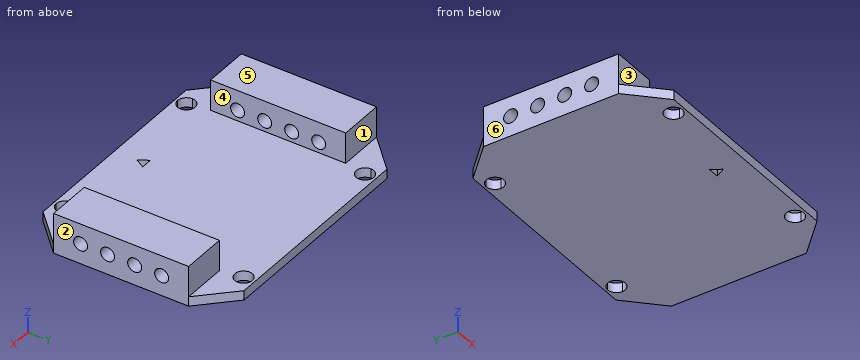
from build123d import *

# Parameters (mm, degrees)
F1_DEPTH = 1.7
F2_W     = 8.1
F2_H     = 24.2000000085
F3_DEPTH = 5.5
F6_DEPTH = 8.1
F7_DEPTH = 8.1


with BuildPart() as f1:
    # F0 (on Top) → F1 (new body)
    with BuildSketch(Plane.XY):
        with BuildLine():
            ThreePointArc((-17.5750000042, 16), (-17.1136931846, 17.1136931804), (-16.0000000042, 17.575))
            Line((-16.0000000042, 17.575), (-16.0000000042, 18))
            Line((-16.0000000042, 18), (-18.8500000085, 18))
            Line((-18.8500000085, 18), (-20.8500000085, 16))
            Line((-20.8500000085, 16), (-17.5750000042, 16))
        make_face()
        with BuildLine():
            ThreePointArc((-16.0000000042, 17.575), (-14.8863068239, 17.1136931804), (-14.4250000042, 16))
            ThreePointArc((-14.4250000042, 16), (-16.0000000042, 14.425), (-17.5750000042, 16))
            Line((-17.5750000042, 16), (-20.8500000085, 16))
            Line((-20.8500000085, 16), (-24.75, 12.1000000085))
            Line((-24.75, 12.1000000085), (-24.75, -12.1))
            Line((-24.75, -12.1), (-20.85, -16))
            Line((-20.85, -16), (-17.5749999958, -16))
            ThreePointArc((-17.5749999958, -16), (-15.9999999958, -14.425), (-14.4249999958, -16))
            ThreePointArc((-14.4249999958, -16), (-14.8863068154, -17.1136931804), (-15.9999999958, -17.575))
            Line((-15.9999999958, -17.575), (-15.9999999958, -18))
            Line((-15.9999999958, -18), (16.0000000042, -18))
            Line((16.0000000042, -18), (16.0000000042, -17.575))
            ThreePointArc((16.0000000042, -17.575), (14.8863068239, -14.8863068196), (17.5750000042, -16))
            Line((17.5750000042, -16), (20.8500000085, -16))
            Line((20.8500000085, -16), (24.75, -12.1000000085))
            Line((24.75, -12.1000000085), (24.75, 12.1))
            Line((24.75, 12.1), (20.85, 16))
            Line((20.85, 16), (17.5749999958, 16))
            ThreePointArc((17.5749999958, 16), (14.8863068154, 14.8863068196), (15.9999999958, 17.575))
            Line((15.9999999958, 17.575), (15.9999999958, 18))
            Line((15.9999999958, 18), (-16.0000000042, 18))
            Line((-16.0000000042, 18), (-16.0000000042, 17.575))
        make_face()
        Polygon((1, -12.2679491924), (0, -14), (-1, -12.2679491924), align=None, mode=Mode.SUBTRACT)
        with BuildLine():
            Line((18.85, 18), (15.9999999958, 18))
            Line((15.9999999958, 18), (15.9999999958, 17.575))
            ThreePointArc((15.9999999958, 17.575), (17.1136931761, 17.1136931804), (17.5749999958, 16))
            Line((17.5749999958, 16), (20.85, 16))
            Line((20.85, 16), (18.85, 18))
        make_face()
        with BuildLine():
            Line((18.8500000085, -18), (20.8500000085, -16))
            Line((20.8500000085, -16), (17.5750000042, -16))
            ThreePointArc((17.5750000042, -16), (17.1136931846, -17.1136931804), (16.0000000042, -17.575))
            Line((16.0000000042, -17.575), (16.0000000042, -18))
            Line((16.0000000042, -18), (18.8500000085, -18))
        make_face()
        with BuildLine():
            Line((-17.5749999958, -16), (-20.85, -16))
            Line((-20.85, -16), (-18.85, -18))
            Line((-18.85, -18), (-15.9999999958, -18))
            Line((-15.9999999958, -18), (-15.9999999958, -17.575))
            ThreePointArc((-15.9999999958, -17.575), (-17.1136931761, -17.1136931804), (-17.5749999958, -16))
        make_face()
    extrude(amount=F1_DEPTH)

    # F2 (on face) → F3 (join)
    with BuildSketch(Plane.XY.offset(1.7)):
        with Locations((-20.7, 4.2e-09)):
            Rectangle(F2_W, F2_H)
        with Locations((20.7, -4.2e-09)):
            Rectangle(F2_W, F2_H)
    extrude(amount=F3_DEPTH)

    # F5 (on face) → F6 (cut)
    with BuildSketch(Plane.YZ.offset(24.75)):
        with BuildLine():
            Line((6.0099999915, 3.6), (8.5099999915, 3.6))
            ThreePointArc((8.5099999915, 3.6), (7.2599999915, 4.85), (6.0099999915, 3.6))
        make_face()
        with BuildLine():
            ThreePointArc((6.0099999915, 3.6), (7.2599999915, 2.35), (8.5099999915, 3.6))
            Line((8.5099999915, 3.6), (6.0099999915, 3.6))
        make_face()
        with BuildLine():
            ThreePointArc((1.1699999915, 3.6), (2.4199999915, 2.35), (3.6699999915, 3.6))
            Line((3.6699999915, 3.6), (1.1699999915, 3.6))
        make_face()
        with BuildLine():
            Line((1.1699999915, 3.6), (3.6699999915, 3.6))
            ThreePointArc((3.6699999915, 3.6), (2.4199999915, 4.85), (1.1699999915, 3.6))
        make_face()
        with BuildLine():
            ThreePointArc((-3.6700000085, 3.6), (-2.4200000085, 2.35), (-1.1700000085, 3.6))
            Line((-1.1700000085, 3.6), (-3.6700000085, 3.6))
        make_face()
        with BuildLine():
            Line((-3.6700000085, 3.6), (-1.1700000085, 3.6))
            ThreePointArc((-1.1700000085, 3.6), (-2.4200000085, 4.85), (-3.6700000085, 3.6))
        make_face()
        with BuildLine():
            Line((-6.0100000085, 3.6), (-8.5100000085, 3.6))
            ThreePointArc((-8.5100000085, 3.6), (-7.2600000085, 2.35), (-6.0100000085, 3.6))
        make_face()
        with BuildLine():
            ThreePointArc((-6.0100000085, 3.6), (-7.2600000085, 4.85), (-8.5100000085, 3.6))
            Line((-8.5100000085, 3.6), (-6.0100000085, 3.6))
        make_face()
    extrude(amount=-F6_DEPTH, mode=Mode.SUBTRACT)

    # F4 (on face) → F7 (cut)
    with BuildSketch(Plane(origin=(-24.75, 0, 0), x_dir=(0, -1, 0), z_dir=(-1, 0, 0))):
        with BuildLine():
            Line((6.0099999915, 3.6), (8.5099999915, 3.6))
            ThreePointArc((8.5099999915, 3.6), (7.2599999915, 4.85), (6.0099999915, 3.6))
        make_face()
        with BuildLine():
            ThreePointArc((6.0099999915, 3.6), (7.2599999915, 2.35), (8.5099999915, 3.6))
            Line((8.5099999915, 3.6), (6.0099999915, 3.6))
        make_face()
        with BuildLine():
            Line((1.1699999915, 3.6), (3.6699999915, 3.6))
            ThreePointArc((3.6699999915, 3.6), (2.4199999915, 4.85), (1.1699999915, 3.6))
        make_face()
        with BuildLine():
            ThreePointArc((1.1699999915, 3.6), (2.4199999915, 2.35), (3.6699999915, 3.6))
            Line((3.6699999915, 3.6), (1.1699999915, 3.6))
        make_face()
        with BuildLine():
            Line((-3.6700000085, 3.6), (-1.1700000085, 3.6))
            ThreePointArc((-1.1700000085, 3.6), (-2.4200000085, 4.85), (-3.6700000085, 3.6))
        make_face()
        with BuildLine():
            ThreePointArc((-3.6700000085, 3.6), (-2.4200000085, 2.35), (-1.1700000085, 3.6))
            Line((-1.1700000085, 3.6), (-3.6700000085, 3.6))
        make_face()
        with BuildLine():
            ThreePointArc((-6.0100000085, 3.6), (-7.2600000085, 4.85), (-8.5100000085, 3.6))
            Line((-8.5100000085, 3.6), (-6.0100000085, 3.6))
        make_face()
        with BuildLine():
            Line((-6.0100000085, 3.6), (-8.5100000085, 3.6))
            ThreePointArc((-8.5100000085, 3.6), (-7.2600000085, 2.35), (-6.0100000085, 3.6))
        make_face()
    extrude(amount=-F7_DEPTH, mode=Mode.SUBTRACT)


solid = f1.part
Could you check a few things on this model? Use its own coordinates, in mm. Face numbers are marked on the shaded views. A direction names the side the tool comes from. Coordinates: 2 decimals unless noted, no trailing zeros. Order: outer loops, then holes, each group sorted by start corner. A loop starts at its lowest first (then second) coordinate and runs counter-clockwise, first axis right, second up. Notation, with made-up numbers: (89, 84.25) - (116, 84.25) arc R15 cw to (116, 103.25) - close; hole circle Ø9 at (26, 60). An arc over 180 degrees is marked (long way). Answer in a Markdown table with one row per item. Add a question column.
(1) I need wall thicknesses on L1, parallel to X at y = -0.5, z = 5; L2, parallel to Z at x = -20.5, y = 7.26; L3, parallel to Z at x = -1.5, y = 13. Which ranges of each line are inside material? Lowest first, please.
(2) Will these pins go through, and if not, where does the flat tip stop? pin 1 (11 mm diameter, centred on x = 9, y = 2, fed in from +Z); pin 2 (3.5 mm diameter, centred on y = 7.26, z = 3.6, fed in from +X); pin 3 (2 mm diameter, centred on y = 2.42, z = 3.6, fed in from -X); pin 4 (1 mm diameter, centred on x = 19, z = 3, fed in from -Y).
(3) On a 3-axis mill with a long thin cutter (end or side, diameter ignored), from which of +Z, -Z, +X, -X, +Y, -Y can I reach the whole of each face in a straight line? I mean the marked faces 1, 2 and 3. Say none if no direction works.
(4) If we section it at D-D, the plane x = 0.5: Please give me the cut outline in (y, z).
(5) If we section it at B-B, the plane z = 5.75: Please give me the cut outline in (x, y).
(6) If we section it at A-A, the plane y = -7.26: Please give me the cut outline in (x, z), then the cut area to 3 significant figures.
(7) If we section it at C-C, the plane x = 15.5: Please give me the cut outline in (y, z).
(8) If we mould it in two halves opening along X, with no side actions, what happens to the marked faces 4, 5 and 6? For each: released by +X, released by -X, zero draft, split by the parting line, or undercut.
Results are:
| question | item | result |
|---|---|---|
| 1 | L1 | x = -24.75 to -16.65, 16.65 to 24.75 |
| 1 | L2 | z = 0 to 2.35, 4.85 to 7.2 |
| 1 | L3 | z = 0 to 1.7 |
| 2 | pin 1 | stops at z = 1.7 |
| 2 | pin 2 | stops at x = 24.75 |
| 2 | pin 3 | passes through |
| 2 | pin 4 | stops at y = -12.1 |
| 3 | face 1 | +Z, +X, -X, +Y |
| 3 | face 2 | +Z, -Z, +X, +Y, -Y |
| 3 | face 3 | +Z, +X, -X, -Y |
| 4 | outline | (-18, 0) - (-13.13, 0) - (-13.13, 1.7) - (-18, 1.7) - close; (-12.27, 0) - (18, 0) - (18, 1.7) - (-12.27, 1.7) - close |
| 5 | outline | (-24.75, -12.1) - (-16.65, -12.1) - (-16.65, 12.1) - (-24.75, 12.1) - close; (16.65, -12.1) - (24.75, -12.1) - (24.75, 12.1) - (16.65, 12.1) - close |
| 6 | outline | (-24.75, 0) - (24.75, 0) - (24.75, 2.35) - (16.65, 2.35) - (16.65, 1.7) - (-16.65, 1.7) - (-16.65, 2.35) - (-24.75, 2.35) - close; (-24.75, 4.85) - (-16.65, 4.85) - (-16.65, 7.2) - (-24.75, 7.2) - close; (16.65, 4.85) - (24.75, 4.85) - (24.75, 7.2) - (16.65, 7.2) - close |
| 6 | area | 133 mm2 |
| 7 | outline | (-18, 0) - (-17.49, 0) - (-17.49, 1.7) - (-18, 1.7) - close; (-14.51, 0) - (14.51, 0) - (14.51, 1.7) - (-14.51, 1.7) - close; (17.49, 0) - (18, 0) - (18, 1.7) - (17.49, 1.7) - close |
| 8 | face 4 | undercut |
| 8 | face 5 | zero draft |
| 8 | face 6 | released by -X |
